from build123d import *

# Parameters (mm, degrees)
CYLINDER063_R     = 4
CYLINDER063_DEPTH = 6
CYLINDER064_R     = 5.5
CYLINDER064_DEPTH = 9
FILLET005_R       = 1
CYLINDER065_R     = 8.9
CYLINDER065_DEPTH = 4


with BuildPart() as cylinder063:
    # Cylinder063 → Cylinder063 (new body)
    with BuildSketch(Plane.XY.offset(15.5)):
        Circle(CYLINDER063_R)
    extrude(amount=CYLINDER063_DEPTH)


with BuildPart() as fillet005:
    # Cylinder064 → Cylinder064 (new body)
    with BuildSketch(Plane.XY.offset(15.5)):
        Circle(CYLINDER064_R)
    extrude(amount=CYLINDER064_DEPTH)

    # Fillet005
    fillet005_edges = [fillet005.edges().sort_by_distance(p)[0] for p in [
        (-5.5, 0, 24.5),
    ]]
    fillet(fillet005_edges, radius=FILLET005_R)


with BuildPart() as hub_cap_middle:
    # Cylinder065 → Cylinder065 (new body)
    with BuildSketch(Plane.XY.offset(15.5)):
        Circle(CYLINDER065_R)
    extrude(amount=CYLINDER065_DEPTH)

    # Fusion031: union Fillet005
    add(fillet005.part)

    # Cut015: cut Cylinder063
    add(cylinder063.part, mode=Mode.SUBTRACT)


solid = hub_cap_middle.part
Source: CAD feature listing. Evaluate the final solid. Frame: model axes, mm. A direction names the side the tool comes from. Give positions to 0.01 mm unless a question says otherwise; leave off trailing zeros. Loops run counter-clockwise (first coordinate to the right, second up) from the corner with the lowest first, then second, coordinate; pieces in that order, holes last. Notation, with made-up numbers: (86.25, -8.5) -> (111.25, -8.5) arc R22 cw to (111.25, 11.5) -> close; hole circle Ø10 at (-31, 55.5). An arc over 180 degrees is marked (long way). Use a Markdown table: item, result. Add a question column.
1) Pull-direction query (Y, two-part tool) for faces 3 (the face through (-0.867, -3.905, 18.458)), 4 (the face through (-1.93, -8.69, 17.47)), 5 (the face through (4, -2, 15.5)), 6 (the face through (0, 0, 21.5)); classes: +Y half, -Y half, draft (parallel to the pull), parting line (faces both ways), or undercut.
2) Section query B-B, the plane z = 20.25. Return the cut outline in (x, y), then the cut area to 3 significant figures.
3) Section query A-A, the plane x = 0. Return the cut outline in (y, z), then the cut area to 3 significant figures.
4) Line query: line 1 along Y through (x, z) = (0, 19); line 2 along Y through (x, z) = (0, 20); line 3 along Z through (x, y) = (6, 2). Output: solid intervals per line, ascending. Write a range as [from, to].
5) Reachability of faces 1 (the face through (-1.19, -5.37, 21.47)), 2 (the face through (0, 0, 24.5)) from +Z, -Z, +X, -X, +Y, -Y: full face, straight path, thin tool, end or side. Return the list, or none.
6) First-contact query: pin 1 (1.5 mm diameter, centred on x = -7, z = 21.5, fed in from -Y); pin 2 (1.5 mm diameter, centred on y = -5, z = 21.5, fed in from +X); pin 3 (2.5 mm diameter, centred on x = 0, y = -0.5, fed in from -Z); pin 4 (1.5 mm diameter, centred on x = -6.5, z = 19, fed in from +Y). Flat tips, straight axial feed; report the tip coordinate or a pass-through.
7) Section query D-D, the plane z = 23. Return the cut outline in (x, y), then the cut area to 3 significant figures.
Numbers:
| question | item | result |
|---|---|---|
| 1 | face 3 | undercut |
| 1 | face 4 | parting line |
| 1 | face 5 | draft |
| 1 | face 6 | undercut |
| 2 | outline | circle Ø11 at (0, 0); hole circle Ø8 at (0, 0) |
| 2 | area | 44.8 mm2 |
| 3 | outline | (-8.9, 15.5) -> (-4, 15.5) -> (-4, 21.5) -> (4, 21.5) -> (4, 15.5) -> (8.9, 15.5) -> (8.9, 19.5) -> (5.5, 19.5) -> (5.5, 23.5) arc R1 ccw to (4.5, 24.5) -> (-4.5, 24.5) arc R1 ccw to (-5.5, 23.5) -> (-5.5, 19.5) -> (-8.9, 19.5) -> close |
| 3 | area | 77.8 mm2 |
| 4 | line 1 | y = [-8.9, -4], [4, 8.9] |
| 4 | line 2 | y = [-5.5, -4], [4, 5.5] |
| 4 | line 3 | z = [15.5, 19.5] |
| 5 | face 1 | +Z |
| 5 | face 2 | +Z, +X, -X, +Y, -Y |
| 6 | pin 1 | passes through |
| 6 | pin 2 | stops at x = 3.49 |
| 6 | pin 3 | stops at z = 21.5 |
| 6 | pin 4 | stops at y = 6.79 |
| 7 | outline | circle Ø11 at (0, 0) |
| 7 | area | 95.0 mm2 |
